```python
from build123d import *

# Parameters (mm, degrees)
SKETCH3_W          = 12.5
SKETCH3_H          = 12.6
CUT_EXTRUDE1_DEPTH = 2.5
CIRPATTERN1_COUNT  = 16
CUT_SWEEP3_ANGLE   = 46.890766
SKETCH8_R          = 27
SKETCH8_R_2        = 19.043703719
CUT_EXTRUDE2_DEPTH = 1.85


# Read off the part's stored shape, not the designer's step: Cut-Sweep3
with BuildPart() as part:
    # Sketch1 → Revolve1 (revolve)
    with BuildSketch(Plane(origin=(0, 0, 0), x_dir=(0, 0, -1), z_dir=(1, 0, 0))):
        Polygon((9.525, 0), (63.5, 0), (63.5, -15), (19.047086271, -15), (19.047086271, -34.735580232), (16.547086271, -34.735580232), (16.547086271, -37.235580232), (19.047086271, -37.235580232), (19.047086271, -40.235580232), (9.525, -40), align=None)
    revolve(axis=Axis((0, 0, 0), (0, 1, 0)))

    # Sketch3 → Cut-Extrude1 (cut)
    with BuildSketch(Plane(origin=(0, 0, 0), x_dir=(1, 0, 0), z_dir=(0, 1, 0))):
        with Locations((0, 50)):
            Rectangle(SKETCH3_W, SKETCH3_H)
    cut_extrude1 = extrude(amount=-CUT_EXTRUDE1_DEPTH, mode=Mode.SUBTRACT)

    # CirPattern1: Cut-Extrude1 ×16 about axis, 2 skipped
    cirpattern1_axis = Axis((0, 0, 0), (0, -1, 0))
    add([cut_extrude1.rotate(cirpattern1_axis, i * 360 / CIRPATTERN1_COUNT) for i in range(1, CIRPATTERN1_COUNT) if i not in (8, 9)], mode=Mode.SUBTRACT)

    # Cut-Sweep3 outline → Cut-Sweep3 (revolve, cut)
    with BuildSketch(Plane(origin=(0, 0, 0), x_dir=(-0.5705578043075055, 0, 0.8212574455941318), z_dir=(-0.8212574455941318, 0, -0.5705578043075055))):
        Polygon((54.406189133, -1.25), (54.406189133, 0), (9.525, 0), (9.525, -13.378851836), align=None)
    revolve(axis=Axis((0, 0, 0), (0, 1, 0)), revolution_arc=CUT_SWEEP3_ANGLE, mode=Mode.SUBTRACT)

    # Sketch8 → Cut-Extrude2 (cut)
    with BuildSketch(Plane.XZ.offset(15)):
        with Locations(Location((0, 0, 0), (0, 0, 270))):
            Circle(SKETCH8_R)
        with Locations(Location((0, 0, 0), (0, 0, 270))):
            Circle(SKETCH8_R_2, mode=Mode.SUBTRACT)
    extrude(amount=-CUT_EXTRUDE2_DEPTH, mode=Mode.SUBTRACT)


solid = part.part
```
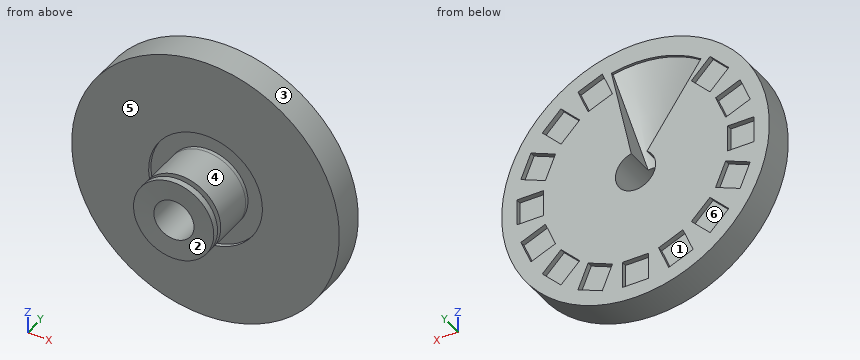
Read the model definition and answer for the solid it produces. Units are mm, in the model's axes. Face numbers are marked on the shaded views. A direction names the side the tool comes from. Round coordinates to 2 decimals unless told otherwise and drop trailing zeros. Write each loop counter-clockwise with the first axis right and the second up, starting at its lowest first coordinate (ties: lowest second). Pieces come first, ordered by that corner, then holes. Notation, with made-up numbers: (-10, 55.25) - (40, 55.25) arc R30 cw to (40, 78.25) - close; hole circle Ø5 at (31, 73). An arc over 180 degrees is marked (long way). Use CSV: the item, a comma, the result in double quotes.
Q1. Determine the mould class of the marked faces 4, 5 and 6 for opening direction X: +X half, -X half, draft (parallel to the pull), parting line (faces both ways), or undercut.
Values:
face 4,"parting line"
face 5,"draft"
face 6,"undercut"
Q2. Each of these flat-tipped pins is pushed along its axis until it touches: pin 1 Ø1.5 at (x, z) = (49.5, 1.5) entering from +Y; pin 2 Ø0.8 at (y, z) = (-1.5, -2) entering from +X; pin 3 Ø1.2 at (x, y) = (49, -1.5) entering from -Z. Where does it stop, or does it pass through?
Values:
pin 1,"stops at y = -2.5"
pin 2,"stops at x = 63.48"
pin 3,"stops at z = -41.11"
Q3. A tool of negligible diameter and unlimited length cuts with its end or side. For the marked faces 1, 2 and 3, from which of +Z, -Z, +X, -X, +Y, -Y can it reach the whole face along a straight path? Write none if from no direction.
Values:
face 1,"+Y"
face 2,"-Y"
face 3,"+Y, -Y"
Q4. Find section D-D, the plane x = -52. Write down the section's boundary in (y, z).
Values:
outline,"(-15, -36.45) - (0, -36.45) - (0, -21.58) - (-2.5, -21.58) - (-2.5, -14.77) - (0, -14.77) - (0, -6.25) - (-2.5, -6.25) - (-2.5, 6.25) - (0, 6.25) - (0, 14.77) - (-2.5, 14.77) - (-2.5, 21.58) - (0, 21.58) - (0, 36.45) - (-15, 36.45) - close"
Q5. Find section B-B, the plane x = 25. Write down the section's boundary in (y, z).
Values:
outline,"(-15, -58.37) - (0, -58.37) - (0, -50.58) - (-2.5, -50.58) - (-2.5, -44.02) - (0, -44.02) - (0, 44.02) - (-2.5, 44.02) - (-2.5, 50.58) - (0, 50.58) - (0, 58.37) - (-15, 58.37) - (-15, 10.2) - (-13.15, 10.2) - (-13.15, -10.2) - (-15, -10.2) - close"
Q6. Find section C-C, the plane z = 56. Write down the section's boundary in (x, y).
Values:
outline,"(-29.94, -15) - (29.94, -15) - (29.94, 0) - (-29.94, 0) - close"
Q7. Straight lines are drawn through the part: line 1 along X through (y, z) = (-14, 0) (3 decimals); line 2 along X through (y, z) = (-10, 0) (3 decimals); line 3 along X through (y, z) = (-30, 0) (3 decimals). For each, find the intervals that lie inside material, in ascending order.
Values:
line 1,"x = -63.5 to -27, -19.044 to -9.525, 9.525 to 19.044, 27 to 63.5"
line 2,"x = -63.5 to -9.525, 9.525 to 63.5"
line 3,"x = -19.047 to -9.525, 9.525 to 19.047"
